```python
from build123d import *

# Parameters (mm, degrees)
F0_W     = 70.000038
F0_H     = 70.000037
F0_R     = 2.9972
F0_R_2   = 2.999994
F0_R_3   = 17.500009
F1_DEPTH = 3.000002


with BuildPart() as f1:
    # F0 (on Top) → F1 (new body)
    with BuildSketch(Plane.XY):
        with Locations((-0.759288, -1.704548)):
            Rectangle(F0_W, F0_H)
        with Locations((-32.000107, -32.945367)):
            Circle(F0_R, mode=Mode.SUBTRACT)
        with Locations((30.481531, -32.945367)):
            Circle(F0_R, mode=Mode.SUBTRACT)
        with Locations((-32.009307, 29.54643)):
            Circle(F0_R_2, mode=Mode.SUBTRACT)
        Circle(F0_R_3, mode=Mode.SUBTRACT)
        with Locations((30.481531, 29.54643)):
            Circle(F0_R_2, mode=Mode.SUBTRACT)
    extrude(amount=F1_DEPTH)


solid = f1.part
```
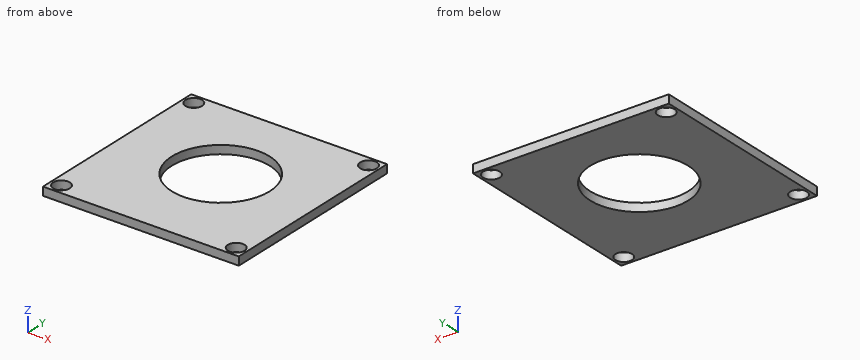
Build history of the part. All positions in model axes, mm. Round coordinates to 2 decimals unless told otherwise and drop trailing zeros. Order: outer loops, then holes, each group sorted by start corner. A loop starts at its lowest first (then second) coordinate and runs counter-clockwise, first axis right, second up. Notation, with made-up numbers: (6, 32) - (54, 32) arc R21 ccw to (54, 56) - close; hole circle Ø6 at (3.25, 38.25). An arc over 180 degrees is marked (long way). Use a Markdown table: item, result.
1) Flat gauge pins, fed straight in: pin 1 Ø1 at (x, y) = (-17.5, -5) entering from -Z; pin 2 Ø3.5 at (x, y) = (30.48, -32.95) entering from -Z. Where does each tip first touch, or does it go through?
Recorded:
| item | result |
|---|---|
| pin 1 | stops at z = 0 |
| pin 2 | passes through |
2) Wall check: L1, parallel to X at y = -1.5, z = 0.85; L2, parallel to Y at x = 15, z = 0.7; L3, parallel to X at y = -11, z = 0.95. Give the ranges that are in metal, low to high.
Recorded:
| item | result |
|---|---|
| L1 | x = -35.76 to -17.44, 17.44 to 34.24 |
| L2 | y = -36.7 to -9.01, 9.01 to 33.3 |
| L3 | x = -35.76 to -13.61, 13.61 to 34.24 |
3) Saw through at A-A on y = 0. Write the cut outline in (x, z), and give its area (3 significant figures).
Recorded:
| item | result |
|---|---|
| outline | (-35.76, 0) - (-17.5, 0) - (-17.5, 3) - (-35.76, 3) - close; (17.5, 0) - (34.24, 0) - (34.24, 3) - (17.5, 3) - close |
| area | 105 mm² |
4) Saw through at C-C on z = 0.85. Write the cut outline in (x, y), and give its area (3 significant figures).
Recorded:
| item | result |
|---|---|
| outline | (-35.76, -36.7) - (34.24, -36.7) - (34.24, 33.3) - (-35.76, 33.3) - close; hole circle Ø6 at (-32.01, 29.55); hole circle Ø5.99 at (-32, -32.95); hole circle Ø35 at (0, 0); hole circle Ø5.99 at (30.48, -32.95); hole circle Ø6 at (30.48, 29.55) |
| area | 3,820 mm² |
5) Saw through at B-B on x = 0. Write the cut outline in (y, z), and give its area (3 significant figures).
Recorded:
| item | result |
|---|---|
| outline | (-36.7, 0) - (-17.5, 0) - (-17.5, 3) - (-36.7, 3) - close; (17.5, 0) - (33.3, 0) - (33.3, 3) - (17.5, 3) - close |
| area | 105 mm² |
